```python
from build123d import *

# Parameters (mm, degrees)
CROQUIS1_W                         = 20
CROQUIS1_H                         = 20
BRIDA_BASE1_DEPTH                  = 1
BRIDA_DE_ARISTA1_STRIP_W           = 5.4732
BRIDA_DE_ARISTA1_STRIP_H           = 1
BRIDA_DE_ARISTA1_STRIP_CUT_DEPTH   = 20
BRIDA_DE_ARISTA1_STRIP_2_W         = 5.4732
BRIDA_DE_ARISTA1_STRIP_2_H         = 1
BRIDA_DE_ARISTA1_STRIP_CUT_2_DEPTH = 20
BRIDA_DE_ARISTA1_DEPTH             = 20
BRIDA_DE_ARISTA1_BEND_DEPTH        = 20
CROQUIS12_R                        = 3
CORTAR_EXTRUIR1_DEPTH              = 35.770677301
REDONDEO1_R                        = 10


# Sheet-metal steps are written as plain solids
with BuildPart() as part:
    # Croquis1 → Brida base1 (new body)
    with BuildSketch(Plane(origin=(0, 0, 0), x_dir=(1, 0, 0), z_dir=(0, 1, 0))):
        Rectangle(CROQUIS1_W, CROQUIS1_H)
    extrude(amount=-BRIDA_BASE1_DEPTH)

    # Brida de arista1 strip (across the edge) → Brida de arista1 strip cut (cut)
    with BuildSketch(Plane(origin=(10, 0, 10), x_dir=(-1, 0, 0), z_dir=(0, 0, -1))):
        with Locations((-2, -0.5)):
            Rectangle(BRIDA_DE_ARISTA1_STRIP_W, BRIDA_DE_ARISTA1_STRIP_H)
    extrude(amount=BRIDA_DE_ARISTA1_STRIP_CUT_DEPTH, mode=Mode.SUBTRACT)

    # Brida de arista1 strip 2 (across the edge) → Brida de arista1 strip cut 2 (cut)
    with BuildSketch(Plane(origin=(-10, 0, -10), x_dir=(1, 0, 0), z_dir=(0, 0, 1))):
        with Locations((-2, -0.5)):
            Rectangle(BRIDA_DE_ARISTA1_STRIP_2_W, BRIDA_DE_ARISTA1_STRIP_2_H)
    extrude(amount=BRIDA_DE_ARISTA1_STRIP_CUT_2_DEPTH, mode=Mode.SUBTRACT)

    # Brida de arista1 section (across the edge) → Brida de arista1 (add)
    with BuildSketch(Plane(origin=(10, 0, 10), x_dir=(-1, 0, 0), z_dir=(0, 0, -1))):
        with BuildLine():
            Line((-1, 0.7366), (-1, 25))
            Line((-1, 25), (0, 25))
            Line((0, 25), (0, 0.7366))
            ThreePointArc((0, 0.7366), (0.215745145, 0.215745145), (0.7366, 0))
            Line((0.7366, 0), (0.7366, -1))
            ThreePointArc((0.7366, -1), (-0.491361636, -0.491361636), (-1, 0.7366))
        make_face()
    extrude(amount=BRIDA_DE_ARISTA1_DEPTH)

    # Brida de arista1 section 2 (across the edge) → Brida de arista1 bend (add)
    with BuildSketch(Plane(origin=(-10, 0, -10), x_dir=(1, 0, 0), z_dir=(0, 0, 1))):
        with BuildLine():
            Line((-1, 0.7366), (-1, 25))
            Line((-1, 25), (0, 25))
            Line((0, 25), (0, 0.7366))
            ThreePointArc((0, 0.7366), (0.215745145, 0.215745145), (0.7366, 0))
            Line((0.7366, 0), (0.7366, -1))
            ThreePointArc((0.7366, -1), (-0.491361636, -0.491361636), (-1, 0.7366))
        make_face()
    extrude(amount=BRIDA_DE_ARISTA1_BEND_DEPTH)

    # Croquis12 → Cortar-Extruir1 (cut, through all)
    with BuildSketch(Plane(origin=(11, 0, 0), x_dir=(0, 0, -1), z_dir=(1, 0, 0))):
        with Locations(Location((0, 18.7366, 0), (0, 0, 90))):
            Circle(CROQUIS12_R)
    extrude(amount=-CORTAR_EXTRUIR1_DEPTH, mode=Mode.SUBTRACT)

    # Redondeo1
    redondeo1_edges = [part.edges().sort_by_distance(p)[0] for p in [
        (-10.5, 25, -10),
        (10.5, 25, -10),
        (10.5, 25, 10),
        (-10.5, 25, 10),
    ]]
    fillet(redondeo1_edges, radius=REDONDEO1_R - 0.0001)  # a hair under: the kernel refuses the full size


solid = part.part
```
Work out the finished part from the listing and answer in its coordinate system (mm). A direction names the side the tool comes from. Coordinates: 2 decimals unless noted, no trailing zeros. Order: outer loops, then holes, each group sorted by start corner. A loop starts at its lowest first (then second) coordinate and runs counter-clockwise, first axis right, second up. Notation, with made-up numbers: (20.5, -16) - (42.5, -16) arc R38 cw to (42.5, 23) - close; hole circle Ø6 at (12, 16). An arc over 180 degrees is marked (long way). Answer as a JSON object with one key per item and string values.
1. A tool of negligible diameter and unlimited length cuts with its end or side. For faces 1 (the face through (10.49, 21.99, -7.15)), 2 (the face through (-10, 13, 0)), from which of +Z, -Z, +X, -X, +Y, -Y can it reach the whole face along a straight path? Write none if from no direction.
Output values:
{"face 1": "-Z, +X, -X, +Y", "face 2": "+Z, -Z, +Y"}
2. Find section C-C on y = 19.25. Determine the outline of the cut face in (x, z).
Output values:
{"outline": "(-11, -9.05) - (-10, -9.05) - (-10, -2.96) - (-11, -2.96) - close; (-11, 2.96) - (-10, 2.96) - (-10, 9.05) - (-11, 9.05) - close; (10, -9.05) - (11, -9.05) - (11, -2.96) - (10, -2.96) - close; (10, 2.96) - (11, 2.96) - (11, 9.05) - (10, 9.05) - close"}
3. Find section B-B on z = 1.75. Determine the outline of the cut face in (x, y).
Output values:
{"outline": "(-11, 0.74) arc R1.74 ccw to (-9.26, -1) - (9.26, -1) arc R1.74 ccw to (11, 0.74) - (11, 16.3) - (10, 16.3) - (10, 0.74) arc R0.74 cw to (9.26, 0) - (-9.26, 0) arc R0.74 cw to (-10, 0.74) - (-10, 16.3) - (-11, 16.3) - close; (-11, 21.17) - (-10, 21.17) - (-10, 24.85) - (-11, 24.85) - close; (10, 21.17) - (11, 21.17) - (11, 24.85) - (10, 24.85) - close"}
4. Find section A-A on y = 9.5. Determine the outline of the cut face in (x, z).
Output values:
{"outline": "(-11, -10) - (-10, -10) - (-10, 10) - (-11, 10) - close; (10, -10) - (11, -10) - (11, 10) - (10, 10) - close"}
5. Each of these flat-tipped pins is pushed along its axis until it touches: P1, Ø8, axis at x = -5, z = -5.5, coming from the +Y side; P2, Ø5, axis at y = 18.74, z = 0, coming from the -X side. Where does it stop, or does it pass through?
Output values:
{"P1": "stops at y = 0", "P2": "passes through"}
6. The mould has two halves that part along Z. Classify faces 3 (the face through (0, 0, 0)), 4 (the face through (10.49, 21.99, 7.15)), 5 (the face through (-10.49, 15.74, 0.13)): +Z half, -Z half, draft (parallel to the pull), parting line (faces both ways), or undercut.
Output values:
{"face 3": "draft", "face 4": "+Z half", "face 5": "undercut"}
7. Consider line 1 (X direction, y = 6, z = 6.25); line 2 (Y direction, x = 1, z = 6.25); line 3 (Y direction, x = 9.75, z = 6.75). Determine where each line is inside the solid, lowest interval first.
Output values:
{"line 1": "x = -11 to -10, 10 to 11", "line 2": "y = -1 to 0", "line 3": "y = -0.93 to 0.18"}
8. Find section D-D on x = -2.75. Determine the outline of the cut face in (y, z), plus the area to 3 significant figures.
Output values:
{"outline": "(-1, -10) - (0, -10) - (0, 10) - (-1, 10) - close", "area": "20.0 mm²"}
